Check sheet for the modelled part. Datum: model origin and axes. Units: mm. Face numbers are marked on the shaded views. A direction names the side the tool comes from. Coordinates: 2 decimals unless noted, no trailing zeros. Write each loop counter-clockwise with the first axis right and the second up, starting at its lowest first coordinate (ties: lowest second). Pieces come first, ordered by that corner, then holes. Notation, with made-up numbers: M 4,36.25 L 15,36.25 A5 ccw 15,44.25 Z; hole C 11.5,-31 d10. An arc over 180 degrees is marked long. Answer as CSV lines item,"result".
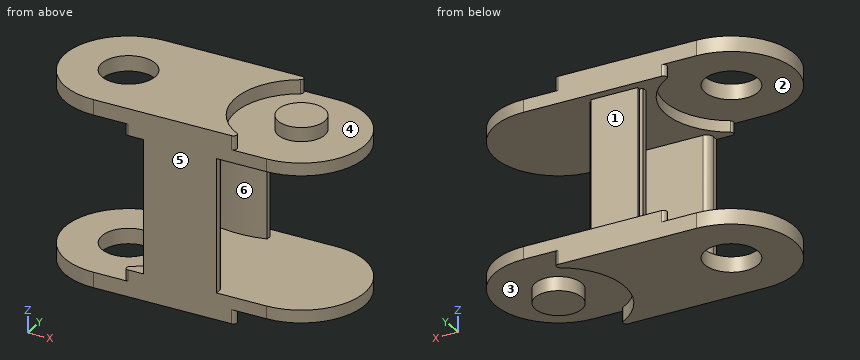
from build123d import *

# Parameters (mm, degrees)
SALIENTE_EXTRUIR1_DEPTH           = 4
CROQUIS2_W                        = 26
CROQUIS2_H                        = 1.9
SALIENTE_EXTRUIR2_DEPTH           = 20
SALIENTE_EXTRUIR3_DEPTH           = 20
SALIENTE_EXTRUIR4_START           = 1.9
SALIENTE_EXTRUIR4_DEPTH           = 1.9
CROQUIS5_W                        = 20
CROQUIS5_H                        = 1.9
CORTAR_EXTRUIR1_DEPTH             = 5.21
CORTAR_EXTRUIR2_START             = -1.7
CORTAR_EXTRUIR2_DEPTH             = 1.7
CROQUIS7_W                        = 20
CROQUIS7_H                        = 1.9
CORTAR_EXTRUIR3_DEPTH             = 2.29
CORTAR_EXTRUIR4_DEPTH             = 20
CORTAR_EXTRUIR5_DEPTH             = 20
CORTAR_EXTRUIR6_DEPTH             = 1.7
CORTAR_EXTRUIR7_START             = -2.1
CORTAR_EXTRUIR7_DEPTH             = 2.1
CROQUIS12_W                       = 20
CROQUIS12_H                       = 1.9
CORTAR_EXTRUIR8_DEPTH             = 7.5
SALIENTE_EXTRUIR5_START           = 2.1
SALIENTE_EXTRUIR5_DEPTH           = 2.1
CROQUIS14_W                       = 3.5
CROQUIS14_H                       = 2.1
CROQUIS15_W                       = 3.5
CROQUIS15_H                       = 2.1
DI_METRO_DE_TALADRO_7_0_7_1_D     = 7
DI_METRO_DE_TALADRO_7_0_7_1_DEPTH = 2.3
DI_METRO_DE_TALADRO_7_0_7_2_D     = 7
DI_METRO_DE_TALADRO_7_0_7_2_DEPTH = 28
NERVIO1_REACH                     = 30.151
CROQUIS20_WALL_W                  = 78.302753042
CROQUIS20_WALL_H                  = 7
REDONDEO1_R                       = 1
CROQUIS21_R                       = 4
CORTAR_EXTRUIR9_DEPTH             = 34


with BuildPart() as part:
    # Croquis1 → Saliente-Extruir1 (new body)
    with BuildSketch(Plane.XY.offset(-10)):
        with BuildLine():
            Line((-13, -9.5), (13, -9.5))
            ThreePointArc((13, -9.5), (22.5, 0), (13, 9.5))
            Line((13, 9.5), (-13, 9.5))
            ThreePointArc((-13, 9.5), (-22.5, 0), (-13, -9.5))
        make_face()
    extrude(amount=-SALIENTE_EXTRUIR1_DEPTH)

    # Croquis2 → Saliente-Extruir2 (add)
    with BuildSketch(Plane.XY.offset(-10)):
        with Locations((0, -8.55)):
            Rectangle(CROQUIS2_W, CROQUIS2_H)
    extrude(amount=SALIENTE_EXTRUIR2_DEPTH)

    # Croquis3 → Saliente-Extruir3 (add)
    with BuildSketch(Plane.XY.offset(-10)):
        with BuildLine():
            Line((-6.2731571, 7.75), (6.2731571, 7.75))
            ThreePointArc((6.2731571, 7.75), (0, 6.4), (-6.2731571, 7.75))
        make_face()
    extrude(amount=SALIENTE_EXTRUIR3_DEPTH)

    # Croquis4 → Saliente-Extruir4 (add)
    with BuildSketch(Plane.XY.offset(10).offset(SALIENTE_EXTRUIR4_START)):
        with BuildLine():
            Line((-13, 9.5), (13, 9.5))
            ThreePointArc((13, 9.5), (22.5, 0), (13, -9.5))
            Line((13, -9.5), (-13, -9.5))
            ThreePointArc((-13, -9.5), (-22.5, 0), (-13, 9.5))
        make_face()
    extrude(amount=-SALIENTE_EXTRUIR4_DEPTH)

    # Croquis5 → Cortar-Extruir1 (cut)
    with BuildSketch(Plane.ZY.offset(13)):
        with Locations((0, -8.55)):
            Rectangle(CROQUIS5_W, CROQUIS5_H)
    extrude(amount=-CORTAR_EXTRUIR1_DEPTH, mode=Mode.SUBTRACT)

    # Croquis6 → Cortar-Extruir2 (cut)
    with BuildSketch(Plane(origin=(0, 0, 10), x_dir=(-1, 0, 0), z_dir=(0, 0, -1)).offset(CORTAR_EXTRUIR2_START)):
        with BuildLine():
            Line((7.79, -9.5), (13, -9.5))
            ThreePointArc((13, -9.5), (22.5, 0), (13, 9.5))
            Line((13, 9.5), (7.79, 9.5))
            ThreePointArc((7.79, 9.5), (8.269213969, 9.142667347), (8.063472742, 8.581415887))
            ThreePointArc((8.063472742, 8.581415887), (3.1, 0), (8.063472742, -8.581415887))
            ThreePointArc((8.063472742, -8.581415887), (8.269213969, -9.142667347), (7.79, -9.5))
        make_face()
    extrude(amount=CORTAR_EXTRUIR2_DEPTH, mode=Mode.SUBTRACT)

    # Croquis7 → Cortar-Extruir3 (cut)
    with BuildSketch(Plane.ZY.offset(7.79)):
        with Locations((0, -8.55)):
            Rectangle(CROQUIS7_W, CROQUIS7_H)
    extrude(amount=-CORTAR_EXTRUIR3_DEPTH, mode=Mode.SUBTRACT)

    # Croquis8 → Cortar-Extruir4 (cut)
    with BuildSketch(Plane(origin=(0, 0, -10), x_dir=(-1, 0, 0), z_dir=(0, 0, -1))):
        with BuildLine():
            Line((4, 7.75), (4, 6.933937347))
            ThreePointArc((4, 6.933937347), (5.152759335, 7.296896808), (6.2731571, 7.75))
            Line((6.2731571, 7.75), (4, 7.75))
        make_face()
    extrude(amount=-CORTAR_EXTRUIR4_DEPTH, mode=Mode.SUBTRACT)

    # Croquis9 → Cortar-Extruir5 (cut)
    with BuildSketch(Plane(origin=(0, 0, -10), x_dir=(-1, 0, 0), z_dir=(0, 0, -1))):
        with BuildLine():
            Line((-4, 6.933937347), (-4, 7.75))
            Line((-4, 7.75), (-6.2731571, 7.75))
            ThreePointArc((-6.2731571, 7.75), (-5.152759335, 7.296896808), (-4, 6.933937347))
        make_face()
    extrude(amount=-CORTAR_EXTRUIR5_DEPTH, mode=Mode.SUBTRACT)

    # Croquis10 → Cortar-Extruir6 (cut)
    with BuildSketch(Plane.XY.offset(-10)):
        with BuildLine():
            Line((-7.79, 9.5), (-13, 9.5))
            ThreePointArc((-13, 9.5), (-22.5, 0), (-13, -9.5))
            Line((-13, -9.5), (-7.79, -9.5))
            ThreePointArc((-7.79, -9.5), (-8.269213969, -9.142667347), (-8.063472742, -8.581415887))
            ThreePointArc((-8.063472742, -8.581415887), (-3.1, 0), (-8.063472742, 8.581415887))
            ThreePointArc((-8.063472742, 8.581415887), (-8.269213969, 9.142667347), (-7.79, 9.5))
        make_face()
    extrude(amount=-CORTAR_EXTRUIR6_DEPTH, mode=Mode.SUBTRACT)

    # Croquis11 → Cortar-Extruir7 (cut)
    with BuildSketch(Plane(origin=(0, 0, -14), x_dir=(-1, 0, 0), z_dir=(0, 0, -1)).offset(CORTAR_EXTRUIR7_START)):
        with BuildLine():
            Line((-13, -9.5), (-7.79, -9.5))
            ThreePointArc((-7.79, -9.5), (-8.269213969, -9.142667347), (-8.063472742, -8.581415887))
            ThreePointArc((-8.063472742, -8.581415887), (-3.1, 0), (-8.063472742, 8.581415887))
            ThreePointArc((-8.063472742, 8.581415887), (-8.269213969, 9.142667347), (-7.79, 9.5))
            Line((-7.79, 9.5), (-13, 9.5))
            ThreePointArc((-13, 9.5), (-22.5, 0), (-13, -9.5))
        make_face()
    extrude(amount=CORTAR_EXTRUIR7_DEPTH, mode=Mode.SUBTRACT)

    # Croquis12 → Cortar-Extruir8 (cut)
    with BuildSketch(Plane(origin=(13, 0, 0), x_dir=(0, 0, -1), z_dir=(1, 0, 0))):
        with Locations((0, -8.55)):
            Rectangle(CROQUIS12_W, CROQUIS12_H)
    extrude(amount=-CORTAR_EXTRUIR8_DEPTH, mode=Mode.SUBTRACT)

    # Croquis13 → Saliente-Extruir5 (add)
    with BuildSketch(Plane.XY.offset(11.9).offset(SALIENTE_EXTRUIR5_START)):
        with BuildLine():
            Line((7.79, -9.5), (-13, -9.5))
            ThreePointArc((-13, -9.5), (-22.5, 0), (-13, 9.5))
            Line((-13, 9.5), (7.79, 9.5))
            ThreePointArc((7.79, 9.5), (8.269213969, 9.142667347), (8.063472742, 8.581415887))
            ThreePointArc((8.063472742, 8.581415887), (3.1, 0), (8.063472742, -8.581415887))
            ThreePointArc((8.063472742, -8.581415887), (8.269213969, -9.142667347), (7.79, -9.5))
        make_face()
    extrude(amount=-SALIENTE_EXTRUIR5_DEPTH)

    # Croquis14 → Revolución1 (revolve)
    with BuildSketch(Plane(origin=(0, 0, 0), x_dir=(1, 0, 0), z_dir=(0, 1, 0))):
        with Locations((14.75, -12.95)):
            Rectangle(CROQUIS14_W, CROQUIS14_H)
    revolve(axis=Axis((13, 0, 11.9), (0, 0, 1)))

    # Croquis15 → Revolución2 (revolve)
    with BuildSketch(Plane.XZ, mode=Mode.PRIVATE) as revoluci_n2_sk:
        with Locations((14.75, -12.95)):
            Rectangle(CROQUIS15_W, CROQUIS15_H)
    revolve(revoluci_n2_sk.sketch.rotate(Axis((13, 0, -11.9), (0, 0, -1)), 180), axis=Axis((13, 0, -11.9), (0, 0, -1)))

    # Diámetro de taladro Ø7.0 (7)1
    with Locations(Plane(origin=(0, 0, 11.7), x_dir=(-1, 0, 0), z_dir=(0, 0, -1))):
        with Locations((13, 0)):
            Hole(DI_METRO_DE_TALADRO_7_0_7_1_D / 2, depth=DI_METRO_DE_TALADRO_7_0_7_1_DEPTH)

    # Diámetro de taladro Ø7.0 (7)2
    with Locations(Plane(origin=(0, 0, -14), x_dir=(-1, 0, 0), z_dir=(0, 0, -1))):
        with Locations((13, 0)):
            Hole(DI_METRO_DE_TALADRO_7_0_7_2_D / 2, depth=DI_METRO_DE_TALADRO_7_0_7_2_DEPTH)

    # Croquis20 wall → Nervio1 (add, up to next)
    with BuildSketch(Plane(origin=(0, 8.25, 0), x_dir=(0, 0, -1), z_dir=(0, -1, 0)), mode=Mode.PRIVATE) as nervio1_sk1:
        Rectangle(CROQUIS20_WALL_W, CROQUIS20_WALL_H)
    nervio1_tool1 = extrude(nervio1_sk1.sketch, amount=NERVIO1_REACH, mode=Mode.PRIVATE) - part.part
    add(nervio1_tool1.solids().sort_by_distance((0, 8.25, 0))[0])

    # Redondeo1
    redondeo1_edges = [part.edges().sort_by_distance(p)[0] for p in [
        (5.5, -7.6, 0),
        (-5.5, -7.6, 0),
    ]]
    fillet(redondeo1_edges, radius=REDONDEO1_R)

    # Croquis21 → Cortar-Extruir9 (cut)
    with BuildSketch(Plane.XY.offset(14)):
        with Locations((-13, 0)):
            Circle(CROQUIS21_R)
    extrude(amount=-CORTAR_EXTRUIR9_DEPTH, mode=Mode.SUBTRACT)


solid = part.part
1) Section check B-B, the plane y = 0. Give the number of separate pieces and of enclosed holes in the cut face, plus the area to 3 significant figures.
Answer key:
separate pieces,"4"
enclosed holes,"0"
area,"205 mm2"
2) Tool access check on the marked faces 1, 2 and 3. Record the directions out of +Z, -Z, +X, -X, +Y, -Y that give a thin tool (end or side, any length) a straight path to the whole face; none if there is none.
Answer key:
face 1,"+X, -X, +Y"
face 2,"-X"
face 3,"-Z"
3) Mould release check, pull along X, two halves, no side actions. Record for the marked faces 4, 5 and 6: pulls with the +X half, pulls with the -X half, needs draft (parallel to the pull), parting line crosses it, or undercut.
Answer key:
face 4,"undercut"
face 5,"needs draft"
face 6,"parting line crosses it"
4) Section check A-A, the plane z = -5. Record the boundary of the cut face in (x, y).
Answer key:
outline,"M -5.5,-9.5 L 5.5,-9.5 L 5.5,-8.6 A1 ccw 4.5,-7.6 L -4.5,-7.6 A1 ccw -5.5,-8.6 Z; M -4,6.93 A15.25 ccw 4,6.93 L 4,7.75 L 3.5,7.75 L 3.5,8.25 L -3.5,8.25 L -3.5,7.75 L -4,7.75 Z"
5) Depth check by flat-ended pin: P1, Ø1, axis at y = 7.5, z = -7.5, coming from the +X side; P2, Ø0.5, axis at y = -9, z = 0, coming from the -X side; P3, Ø7.5, axis at x = -1, z = -2, coming from the +Y side; P4, Ø1, axis at x = -15, y = -2, coming from the -Z side. Enter the tip coordinate at first touch or a pass-through.
Answer key:
P1,"stops at x = 4"
P2,"stops at x = -5.5"
P3,"stops at y = 8.25"
P4,"passes through"
6) Section check D-D, the plane x = -16.5. Record the boundary of the cut face in (y, z), plus the area to 3 significant figures.
Answer key:
outline,"M -8.83,-14 L -1.94,-14 L -1.94,-11.7 L -8.83,-11.7 Z; M -8.83,11.7 L -1.94,11.7 L -1.94,14 L -8.83,14 Z; M 1.94,-14 L 8.83,-14 L 8.83,-11.7 L 1.94,-11.7 Z; M 1.94,11.7 L 8.83,11.7 L 8.83,14 L 1.94,14 Z"
area,"63.4 mm2"
7) Section check C-C, the plane y = -7. Record the boundary of the cut face in (x, z).
Answer key:
outline,"M -19.42,-14 L 6,-14 L 6,-11.9 L 19.42,-11.9 L 19.42,-10 L -6,-10 L -6,-11.7 L -19.42,-11.7 Z; M -19.42,11.7 L -6,11.7 L -6,10 L 19.42,10 L 19.42,11.9 L 6,11.9 L 6,14 L -19.42,14 Z"
8) Thickness scan on line 1 along Z through (x, y) = (-15.5, -5.75); line 2 along Y through (x, z) = (-13, 13.1); line 3 along Z through (x, y) = (8, -8.5). Record the ranges inside material, lowest first.
Answer key:
line 1,"z = -14 to -11.7, 11.7 to 14"
line 2,"y = -9.5 to -4, 4 to 9.5"
line 3,"z = -11.9 to -10, 10 to 11.9"
